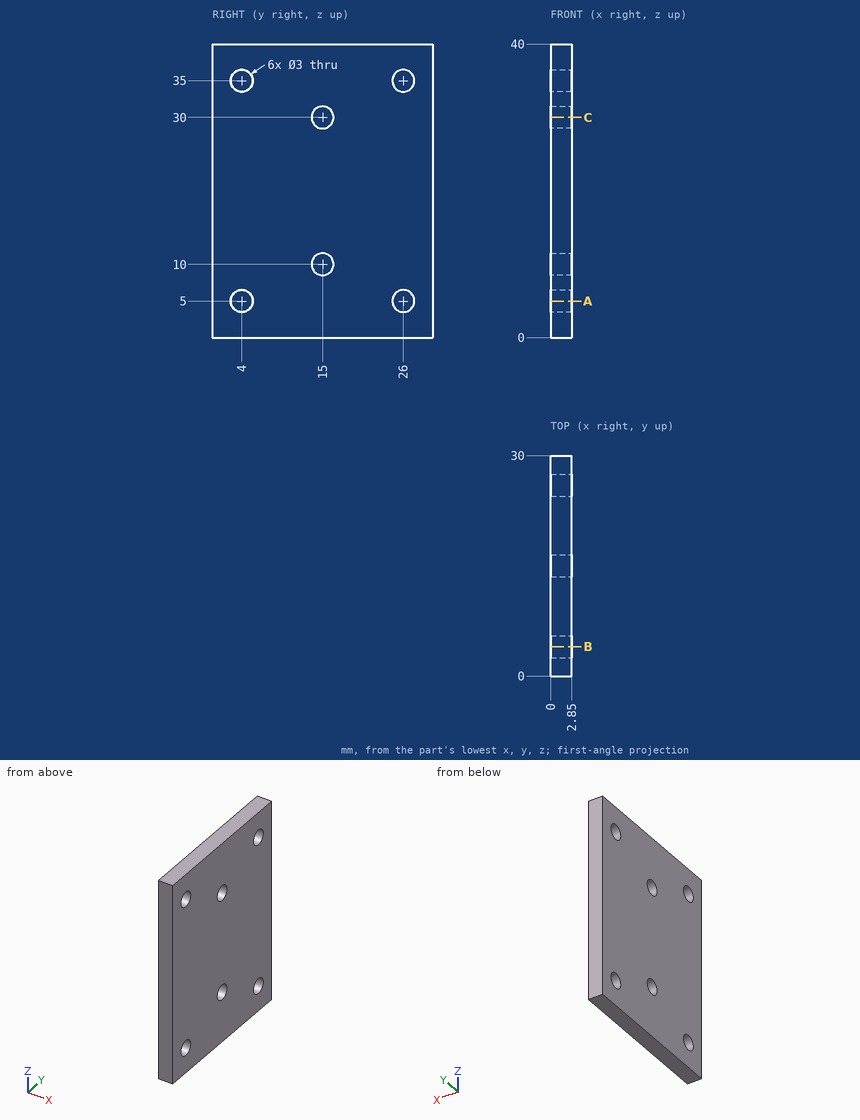
Source: three-view drawing plus pictorial views. Frame: mm from the lowest corner of the part. Coordinates: 2 decimals unless noted, no trailing zeros. Order: outer loops, then holes, each group sorted by start corner. A loop starts at its lowest first (then second) coordinate and runs counter-clockwise, first axis right, second up. Notation, with made-up numbers: M 46.5,69.5 L 63.5,69.5 A29 ccw 63.5,106.5 Z; hole C 89.25,17 d10. An arc over 180 degrees is marked long. One line per question, with ' | ' between items.
Item 1: Pin query (flat end, axial travel): pin 1 (1.8 mm diameter, centred on y = 4, z = 5, fed in from -X). Return the tip coordinate at first contact, or that it passes through.
Geometry results:
pin 1: passes through
Item 2: Section A-A (z = 5). Output: boundary loops of the cut face in (x, y).
Geometry results:
outline: M 0,0 L 2.85,0 L 2.85,2.5 L 0,2.5 Z; M 0,5.5 L 2.85,5.5 L 2.85,24.5 L 0,24.5 Z; M 0,27.5 L 2.85,27.5 L 2.85,30 L 0,30 Z
Item 3: Ray query, line 1 along Y through (x, z) = (0.8, 5); line 2 along Y through (x, z) = (2.4, 36); line 3 along Z through (x, y) = (1.7, 26.25). Return the intervals inside material, ascending.
Geometry results:
line 1: y = 0 to 2.5, 5.5 to 24.5, 27.5 to 30 | line 2: y = 0 to 2.88, 5.12 to 24.88, 27.12 to 30 | line 3: z = 0 to 3.52, 6.48 to 33.52, 36.48 to 40
Item 4: Section C-C (z = 30). Output: boundary loops of the cut face in (x, y).
Geometry results:
outline: M 0,0 L 2.85,0 L 2.85,13.5 L 0,13.5 Z; M 0,16.5 L 2.85,16.5 L 2.85,30 L 0,30 Z
Item 5: Section B-B (y = 4). Output: boundary loops of the cut face in (x, z), then the cut area to 3 significant figures.
Geometry results:
outline: M 0,0 L 2.85,0 L 2.85,3.5 L 0,3.5 Z; M 0,6.5 L 2.85,6.5 L 2.85,33.5 L 0,33.5 Z; M 0,36.5 L 2.85,36.5 L 2.85,40 L 0,40 Z | area: 96.9 mm^2
